Can you work these out from the drawing? Everything is in mm from the part's minimum corner. A direction names the side the tool comes from. Give positions to 0.01 mm unless a question says otherwise; leave off trailing zeros. Order: outer loops, then holes, each group sorted by start corner. A loop starts at its lowest first (then second) coordinate and runs counter-clockwise, first axis right, second up. Notation, with made-up numbers: M 47,-29.5 L 104,-29.5 A15 ccw 104,-14.5 Z; hole C 85.5,-21 d8. An arc over 180 degrees is marked long. Use a Markdown table: item, result. Add a question column.
Item 1: If I drill on L1, parallel to X at y = 15.5, z = 18; L2, parallel to X at y = 1.75, z = 7.25 (1 decimal); L3, parallel to Y at x = 19, z = 17.75, over which ranges is the centre line in solid material (lowest first)? Write a range as from..to.
Item 2: Suppose I cut it at C-C on z = 17. Write out the boundary of the cut face in (x, y), plus the area to 3 significant figures.
Item 3: If we mould it in two halves opening along X, with no side actions, what happens to the marked faces 4, 5 and 6? For each: released by +X, released by -X, zero draft, split by the parting line, or undercut.
Item 4: Suppose I cut it at A-A on x = 20. Write out the boundary of the cut face in (y, z), plus the area to 3 significant figures.
Item 5: Suppose I cut it at B-B on y = 12.5. Write out the boundary of the cut face in (x, z), plus the area to 3 significant figures.
Item 6: Suppose I cut it at D-D on x = 48.5. Write out the boundary of the cut face in (y, z), plus the area to 3 significant figures.
Item 7: For the marked faces 1, 2 and 3, which set-ups out of +Z, -Z, +X, -X, +Y, -Y let a thin tool reach every point of the face, with its end or its side?
Item 8: I'm going to push flat-ended pins straight in: pin 1 Ø1.8 at (y, z) = (11, 16.5) entering from -X; pin 2 Ø4 at (x, y) = (18, 14.5) entering from +Z; pin 3 Ø6 at (x, y) = (11, 13) entering from -Z; pin 4 Ø6.5 at (y, z) = (12, 18) entering from +X. Where does each tip first touch, or does it pass through?
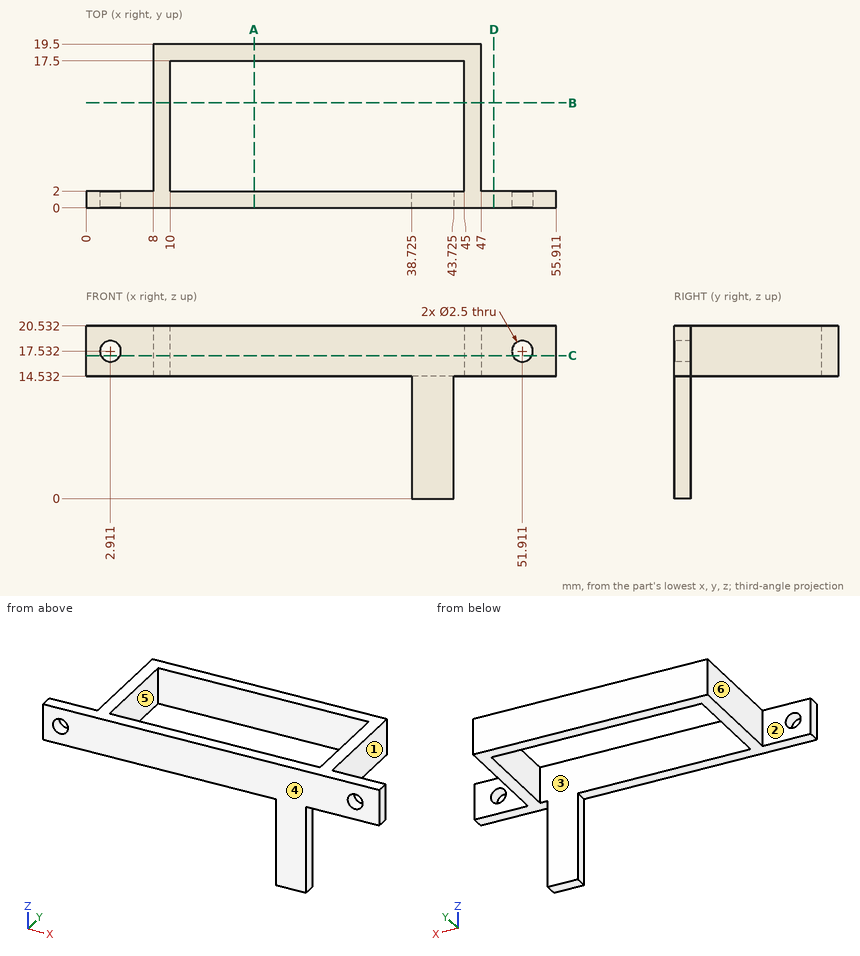
Findings below:
| question | item | result |
|---|---|---|
| 1 | L1 | x = 8..10, 45..47 |
| 1 | L2 | x = 38.7..43.7 |
| 1 | L3 | y = 0..2, 17.5..19.5 |
| 2 | outline | M 0,0 L 1.78,0 L 1.78,2 L 0,2 Z; M 4.04,0 L 50.78,0 L 50.78,2 L 47,2 L 47,19.5 L 8,19.5 L 8,2 L 4.04,2 Z; M 53.04,0 L 55.91,0 L 55.91,2 L 53.04,2 Z; hole M 10,2 L 45,2 L 45,17.5 L 10,17.5 Z |
| 2 | area | 243 mm^2 |
| 3 | face 4 | zero draft |
| 3 | face 5 | undercut |
| 3 | face 6 | released by -X |
| 4 | outline | M 0,14.53 L 2,14.53 L 2,20.53 L 0,20.53 Z; M 17.5,14.53 L 19.5,14.53 L 19.5,20.53 L 17.5,20.53 Z |
| 4 | area | 24.0 mm^2 |
| 5 | outline | M 8,14.53 L 10,14.53 L 10,20.53 L 8,20.53 Z; M 45,14.53 L 47,14.53 L 47,20.53 L 45,20.53 Z |
| 5 | area | 24.0 mm^2 |
| 6 | outline | M 0,14.53 L 2,14.53 L 2,20.53 L 0,20.53 Z |
| 6 | area | 12.0 mm^2 |
| 7 | face 1 | +Z, -Z, +X, +Y |
| 7 | face 2 | +Z, -Z, -X, +Y |
| 7 | face 3 | +Z, -Z |
| 8 | pin 1 | stops at x = 8 |
| 8 | pin 2 | passes through |
| 8 | pin 3 | stops at z = 14.53 |
| 8 | pin 4 | stops at x = 47 |
